Input: part model. Units: mm. Frame: model coordinates. A direction names the side the tool comes from. Give positions to 0.01 mm unless a question says otherwise; leave off trailing zeros. Loops run counter-clockwise (first coordinate to the right, second up) from the corner with the lowest first, then second, coordinate; pieces in that order, holes last. Notation, with made-up numbers: (54.25, 68.5) - (98.25, 68.5) arc R14 ccw to (98.25, 72.5) - close; hole circle Ø11 at (-33.5, -2.5). An arc over 180 degrees is marked (long way). One line per item, written item: value.
from build123d import *

# Parameters (mm, degrees)
F0_W     = 609.6
F0_H     = 914.4
F1_DEPTH = 263.525
F2_T     = -12.7
F3_W     = 584.2
F3_H     = 19.05
F4_DEPTH = 250.825
F5_W     = 584.2
F5_H     = 19.05
F6_DEPTH = 250.825


# Not quite as in the source:
# - the program builds the solid bodies; features that only make, move or delete a surface that nothing else refers to are left out


with BuildPart() as f1:
    # F0 (on Front) → F1 (new body)
    with BuildSketch(Plane.XZ):
        Rectangle(F0_W, F0_H)
    extrude(amount=F1_DEPTH)

    # F2
    f2_openings = [f1.faces().sort_by_distance(p)[0] for p in [
        (0, -263.525, 0),
    ]]
    offset(amount=F2_T, openings=f2_openings)

    # F3 (on face) → F4 (join)
    with BuildSketch(Plane.XZ.offset(12.7)):
        with Locations((0, -180.975)):
            Rectangle(F3_W, F3_H)
    extrude(amount=F4_DEPTH)

    # F5 (on face) → F6 (join)
    with BuildSketch(Plane.XZ.offset(12.7)):
        with Locations((0, 13.335)):
            Rectangle(F5_W, F5_H)
        with Locations((0, 243.205)):
            Rectangle(F5_W, F5_H)
    extrude(amount=F6_DEPTH)


solid = f1.part
Item 1: Section B-B, the plane z = -159.5. Output: boundary loops of the cut face in (x, y) (3 decimals).
Verdict:
outline: (-304.8, -263.525) - (-292.1, -263.525) - (-292.1, -12.7) - (292.1, -12.7) - (292.1, -263.525) - (304.8, -263.525) - (304.8, 0) - (-304.8, 0) - close
Item 2: Section A-A, the plane y = -179. Output: boundary loops of the cut face in (x, z).
Verdict:
outline: (-304.8, -457.2) - (304.8, -457.2) - (304.8, 457.2) - (-304.8, 457.2) - close; hole (-292.1, -444.5) - (292.1, -444.5) - (292.1, -190.5) - (-292.1, -190.5) - close; hole (-292.1, -171.45) - (292.1, -171.45) - (292.1, 3.81) - (-292.1, 3.81) - close; hole (-292.1, 22.86) - (292.1, 22.86) - (292.1, 233.68) - (-292.1, 233.68) - close; hole (-292.1, 252.73) - (292.1, 252.73) - (292.1, 444.5) - (-292.1, 444.5) - close
Item 3: Draft query along Z for faces 3 (the face through (-4, -130, -457.2)), 4 (the face through (304.8, -130, -6)), 5 (the face through (-4, -136, 22.86)). Return one class per face: pulls with the +Z half, pulls with the -Z half, needs draft (parallel to the pull), parting line crosses it, or undercut.
Verdict:
face 3: pulls with the -Z half
face 4: needs draft
face 5: undercut
Item 4: Access query for faces 1 (the face through (-137, -263.525, 239)), 2 (the face through (-292.1, -136, 127)). Directions: +Z, -Z, +X, -X, +Y, -Y. A direction counts if a zero-diameter tool reaches every point of the face in a straight line with its end or side. Return the directions, or none.
Verdict:
face 1: +Z, -Z, +X, -X, -Y
face 2: -Y
Item 5: Section C-C, the plane x = 4. Output: boundary loops of the cut face in (y, z) (3 decimals).
Verdict:
outline: (-263.525, -457.2) - (0, -457.2) - (0, 457.2) - (-263.525, 457.2) - (-263.525, 444.5) - (-12.7, 444.5) - (-12.7, 252.73) - (-263.525, 252.73) - (-263.525, 233.68) - (-12.7, 233.68) - (-12.7, 22.86) - (-263.525, 22.86) - (-263.525, 3.81) - (-12.7, 3.81) - (-12.7, -171.45) - (-263.525, -171.45) - (-263.525, -190.5) - (-12.7, -190.5) - (-12.7, -444.5) - (-263.525, -444.5) - close
Item 6: Pin query (flat end, axial travel): P1, Ø4, axis at x = 167, z = -228.5, coming from the -Y side. Return the tip coordinate at first contact, or that it passes through.
Verdict:
P1: stops at y = -12.7
Item 7: Material intervals for L1, parallel to Z at x = 89.5, y = -133; L2, parallel to X at y = -129, z = 363.5; L3, parallel to Y at x = -135, z = -274.5, sorted ascending.
Verdict:
L1: z = -457.2 to -444.5, -190.5 to -171.45, 3.81 to 22.86, 233.68 to 252.73, 444.5 to 457.2
L2: x = -304.8 to -292.1, 292.1 to 304.8
L3: y = -12.7 to 0
